Study the drawing (mm; zero at the part's minimum x, y, z) and answer. Coordinates: 2 decimals unless noted, no trailing zeros. Loops run counter-clockwise (first coordinate to the right, second up) from the corner with the lowest first, then second, coordinate; pieces in that order, holes last. Notation, with made-up numbers: (16.5, -12.5) - (28.5, -12.5) arc R10 cw to (28.5, 1.5) - close; hole circle Ø6 at (53, 11). An arc over 180 degrees is marked (long way). Use one line per item in the form item = value. Start each with the question number.
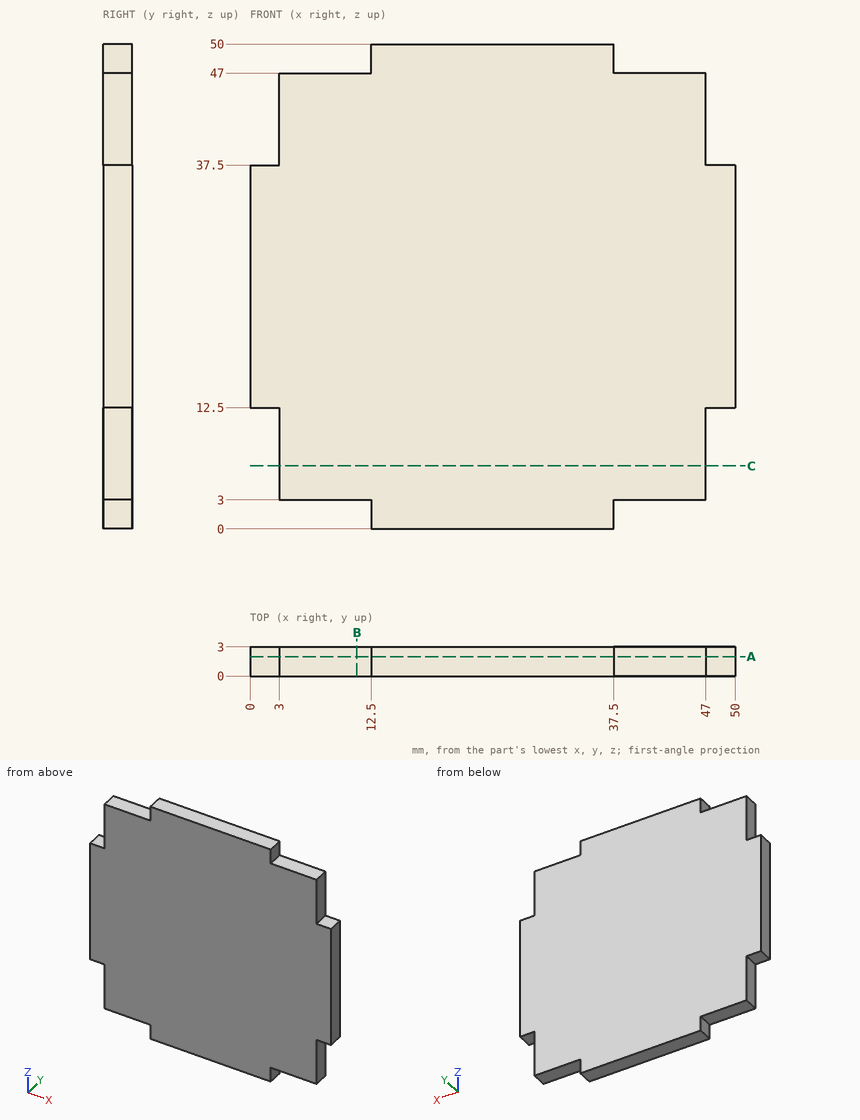
(1) A cutting plane is placed at C-C (z = 6.5). Determine the outline of the cut face in (x, y), then the cut area to 3 significant figures.
(2) Find the intervals of material crossed by probe 1 along Z at (x, y) = (7, 2.4); probe 2 along Z at (x, y) = (2.5, 2.6), in increasing order. Write a range as from..to.
(3) A cutting plane is placed at A-A (y = 2). Determine the outline of the cut face in (x, z), then the cut area to 3 significant figures.
(4) A cutting plane is placed at B-B (x = 11). Determine the outline of the cut face in (y, z).
(5) Each of these flat-tipped pins is pushed along its axis until it touches: pin 1 Ø1.5 at (y, z) = (1, 39) entering from +X; pin 2 Ø1 at (x, z) = (7, 5) entering from -Y; pin 3 Ø0.9 at (x, y) = (49, 1) entering from -Z; pin 4 Ø1.5 at (y, z) = (2, 2) entering from -X. Where does it stop, or does it pass through?
Evaluation:
q1.outline = (3, 0) - (47, 0) - (47, 3) - (3, 3) - close
q1.area = 132 mm^2
q2.probe_1 = 3..47
q2.probe_2 = 12.5..37.5
q3.outline = (0, 12.5) - (3, 12.5) - (3, 3) - (12.5, 3) - (12.5, 0) - (37.5, 0) - (37.5, 3) - (47, 3) - (47, 12.5) - (50, 12.5) - (50, 37.5) - (47, 37.5) - (47, 47) - (37.5, 47) - (37.5, 50) - (12.5, 50) - (12.5, 47) - (3, 47) - (3, 37.5) - (0, 37.5) - close
q3.area = 2,240 mm^2
q4.outline = (0, 3) - (3, 3) - (3, 47) - (0, 47) - close
q5.pin_1 = 47
q5.pin_2 = 0
q5.pin_3 = 12.5
q5.pin_4 = 12.5
